Autodesk Inventor part; units mm, degrees
ref_plane "YZ Plane" through (0, 0, 0) normal (1, 0, 0) x (0, 1, 0)
ref_plane "XZ Plane" through (0, 0, 0) normal (0, 1, 0) x (-1, 0, 0)
ref_plane "XY Plane" through (0, 0, 0) normal (0, 0, 1) x (1, 0, 0)
sketch "Skizze1" plane through (0, 0, 0) normal (0, 1, 0) x (-1, 0, 0)
  line L0 (0, 0) -> (0, 74)
  line L1 (0, 74) -> (16, 74)
  line L2 (16, 74) -> (16, 44)
  line L3 (16, 44) -> (192, 44)
  arc A0 (192, -44) -> (192, 44) centre (192, 0) ccw
  line L4 (192, -44) -> (16, -44)
  line L5 (16, -44) -> (16, -74)
  line L6 (16, -74) -> (0, -74)
  line L7 (0, -74) -> (0, 0)
  line L8 (0, 0) -> (236, 0) construction
  dimension "d0" = 192
  dimension "d1" = 16
  dimension "d2" = 30
  dimension "d3" = 44
extrude "Extrusion1" add sketch "Skizze1" along normal blind 24
sketch "Skizze2" plane through (0, 24, 0) normal (0, 1, 0) x (1, 0, 0)
  arc A0 (-192, 44) -> (-192, -44) centre (-192, 0) ccw
  point P0 (0, 0)
hole "Bohrung1" at (-192, 24, 0) direction (0, -1, 0) diameter 60 depth 18
sketch "Skizze3" plane through (-192, 6, 0) normal (0, 1, 0) x (1, 0, 0)
  circle A0 centre (0, 0) radius 30
  point P0 (192, 0)
hole "Bohrung2" at (-192, 6, 0) direction (0, -1, 0) diameter 28 depth 6
sketch "Skizze4" plane through (0, 24, 0) normal (0, 1, 0) x (1, 0, 0)
  line L0 (-40, 0) -> (-128, 0) construction
  line L1 (-40, 24) -> (-128, 24)
  line L2 (-128, -24) -> (-40, -24)
  arc A0 (-40, -24) -> (-40, 24) centre (-40, 0) ccw
  arc A1 (-128, 24) -> (-128, -24) centre (-128, 0) ccw
  line L3 (0, -74) -> (0, 74)
  line L4 (-16, -44) -> (-16, -74)
  point P0 (0, 0)
  point P1 (-84, 0)
  point P2 (0, 0)
  point P3 (0, 0)
  dimension "d20" = 88
  dimension "d21" = 48
  dimension "d22" = 24
extrude "Extrusion2" cut sketch "Skizze4" against normal up to surface (24 mm away)
sketch "Skizze5" plane through (-16, 0, -74) normal (-1, 0, 0) x (0, 0, 1)
  line L0 (148, 0) -> (148, 24)
  line L1 (0, 0) -> (0, 24)
  point P0 (74, 0)
  point P1 (14, 12)
  point P2 (134, 12)
  point P3 (148, 12)
  point P4 (0, 12)
  dimension "d32" = 120
  dimension "d33" = 60
hole "Bohrung3" at (-16, 12, -60) at (-16, 12, 60) direction (1, 0, 0) diameter 12 depth 16
properties part number "1" material "Messing, weicher Gelbton"
Read the model definition and answer for the solid it produces. Units are mm, in the model's axes. A direction names the side the tool comes from. Round coordinates to 2 decimals unless told otherwise and drop trailing zeros. Write each loop counter-clockwise with the first axis right and the second up, starting at its lowest first coordinate (ties: lowest second). Pieces come first, ordered by that corner, then holes. Notation, with made-up numbers: (-25.5, 46.25) - (22.5, 46.25) arc R20 ccw to (22.5, 78.25) - close; hole circle Ø4 at (-31.75, 55). An arc over 180 degrees is marked (long way). One line per question, with ' | ' between items. Start each with the question number.
1. Section B-B (y = 12) is taken. Determine the outline of the cut face in (x, z).
2. Find the intervals of material crossed by probe 1 along X at (y, z) = (2.85, 0); probe 2 along Z at (x, y) = (-80, 7); probe 3 along Z at (x, y) = (-8, 12), in increasing order. Write a range as [from, to].
3. For a pull along Y with two mould halves and no side action, classify faces 4 (the face through (-8, 12, -66)), 5 (the face through (-105, 12, -44)), 6 (the face through (-186, 6, 13)) as +Y half, -Y half, draft (parallel to the pull), parting line (faces both ways), or undercut.
4. Each of these flat-tipped pins is pushed along its axis until it touches: pin 1 (9.5 mm diameter, centred on y = 12, z = 60, fed in from +X); pin 2 (1.5 mm diameter, centred on x = -211.5, z = -9, fed in from +Y); pin 3 (12 mm diameter, centred on x = -131, y = 11, fed in from +Z); pin 4 (12 mm diameter, centred on y = 5.5, z = 57, fed in from -X). Where does it stop, or does it pass through?
5. Section C-C (x = -98) is taken. Determine the outline of the cut face in (y, z).
6. Section A-A (z = 0) is taken. Determine the outline of the cut face in (x, y).
7. Section D-D (z = 60) is taken. Determine the outline of the cut face in (x, y), and give its area (3 significant figures).
8. For faces 1 (the face through (-16, 6, 56)), 2 (the face through (-16.006, 12.168, 0.528)), 3 (the face through (-16, 6, -55)), determine the directions among +Z, -Z, +X, -X, +Y, -Y from which every point of the face is accessible in a straight line to the end or side of a thin tool.
Filled in:
1) outline: (-192, -44) - (-16, -44) - (-16, -54) - (0, -54) - (0, 54) - (-16, 54) - (-16, 44) - (-192, 44) arc R44 ccw to start; (-16, -74) - (0, -74) - (0, -66) - (-16, -66) - close; (-16, 66) - (0, 66) - (0, 74) - (-16, 74) - close; hole circle Ø60 at (-192, 0); hole (-128, -24) - (-40, -24) arc R24 ccw to (-40, 24) - (-128, 24) arc R24 ccw to start
2) probe 1: [-236, -206], [-178, -152], [-16, 0] | probe 2: [-44, -24], [24, 44] | probe 3: [-74, -66], [-54, 54], [66, 74]
3) face 4: undercut | face 5: draft | face 6: +Y half
4) pin 1: through | pin 2: y = 6 | pin 3: z = 44 | pin 4: x = -16
5) outline: (0, -44) - (24, -44) - (24, -24) - (0, -24) - close; (0, 24) - (24, 24) - (24, 44) - (0, 44) - close
6) outline: (-236, 0) - (-206, 0) - (-206, 6) - (-222, 6) - (-222, 24) - (-236, 24) - close; (-178, 0) - (-152, 0) - (-152, 24) - (-162, 24) - (-162, 6) - (-178, 6) - close; (-16, 0) - (0, 0) - (0, 24) - (-16, 24) - close
7) outline: (-16, 0) - (0, 0) - (0, 6) - (-16, 6) - close; (-16, 18) - (0, 18) - (0, 24) - (-16, 24) - close | area: 192 mm²
8) face 1: +Z, -X, +Y, -Y | face 2: +Y, -Y | face 3: -Z, -X, +Y, -Y
